Here's the drawing with two shaded views (mm, measured from the low corner). I have some questions. Coordinates: 2 decimals unless noted, no trailing zeros. Write each loop counter-clockwise with the first axis right and the second up, starting at its lowest first coordinate (ties: lowest second). Pieces come first, ordered by that corner, then holes. Notation, with made-up numbers: (58, 63.5) -> (62, 63.5) arc R18 ccw to (62, 92.5) -> close; hole circle Ø7 at (53, -7.75). An arc over 180 degrees is marked (long way). Put each result on its own line as item: value. Start each with the question number.
Item 1: I want a section at A-A, the plane x = 43. List the corners of the cut face in (y, z) for me (1 decimal).
Item 2: If we mould it in two halves opening along X, with no side actions, what happens to the marked faces 1, 2 and 3? For each: released by +X, released by -X, zero draft, split by the parting line, or undercut.
Item 3: I want a section at C-C, the plane z = 16. List the corners of the cut face in (x, y) for me (1 decimal).
Item 4: I need wall thicknesses on line 1 (X direction, y = 2.25, z = 43) (1 decimal); line 2 (Z direction, x = 39.5, y = 0.7) (1 decimal). Which ranges of each line are inside material? Lowest first, please. Write a range as [from, to].
Item 5: I want a section at B-B, the plane z = 43. List the corners of the cut face in (x, y) for me (1 decimal).
Item 6: I want a section at D-D, the plane x = 61. List the corners of the cut face in (y, z) for me (1 decimal), then the cut area to 3 significant figures.
Item 7: For pin 1 (1.6 mm diameter, centred on x = 50, y = 1.5, fed in from -Z); pin 2 (5 mm diameter, centred on x = 73.5, z = 28, fed in from +Y), each with a flat end and sliding along its axis, tell me the tip position at first contact or that it passes through.
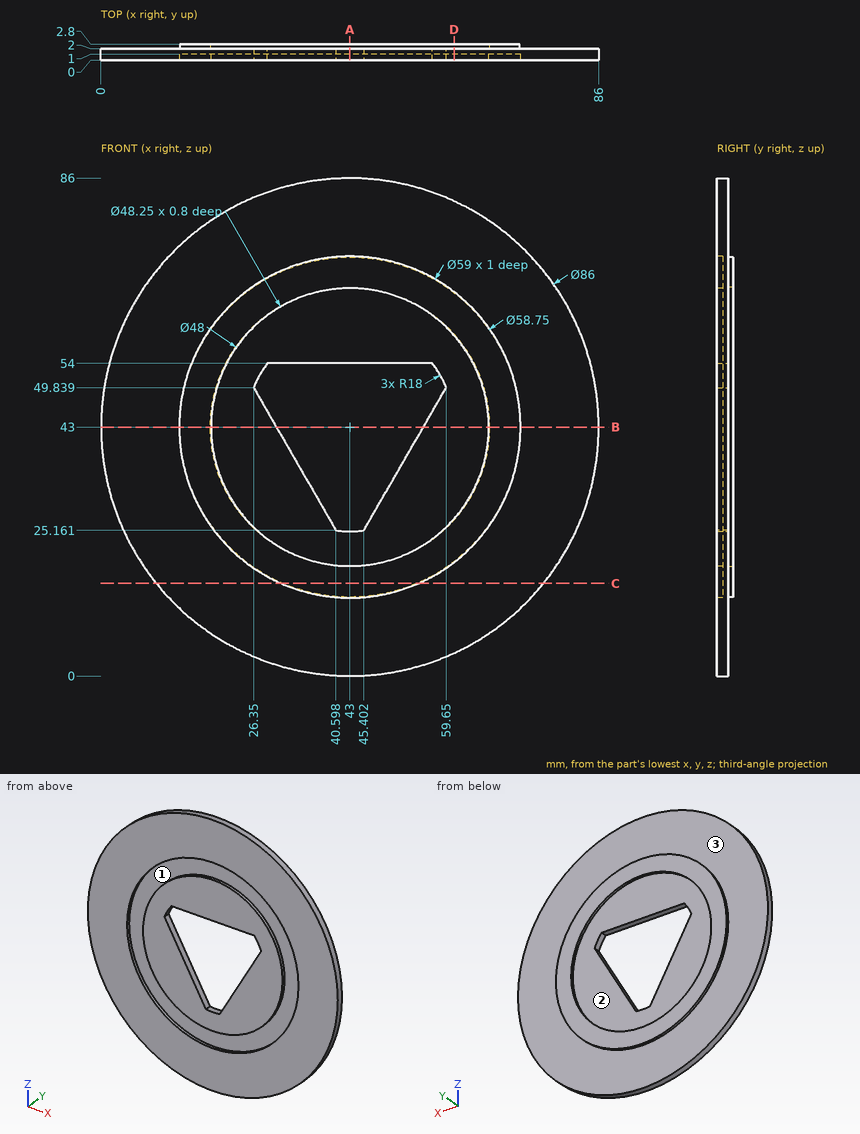
Calculated:
1. outline: (0, 0) -> (2, 0) -> (2, 13.6) -> (2.8, 13.6) -> (2.8, 18.9) -> (2, 18.9) -> (2, 25) -> (0, 25) -> (0, 19) -> (1, 19) -> (1, 13.5) -> (0, 13.5) -> close; (0, 54) -> (2, 54) -> (2, 67.1) -> (2.8, 67.1) -> (2.8, 72.4) -> (2, 72.4) -> (2, 86) -> (0, 86) -> (0, 72.5) -> (1, 72.5) -> (1, 67) -> (0, 67) -> close
2. face 1: undercut
2. face 2: undercut
2. face 3: zero draft
3. outline: (9.5, 0) -> (31.1, 0) -> (31.1, 1) -> (54.9, 1) -> (54.9, 0) -> (76.5, 0) -> (76.5, 2) -> (54.6, 2) -> (54.6, 2.8) -> (31.4, 2.8) -> (31.4, 2) -> (9.5, 2) -> close
4. line 1: x = [13.6, 18.9], [67.1, 72.4]
4. line 2: z = [0.1, 13.7], [19.3, 27.1], [54, 66.7], [72.3, 85.9]
5. outline: (0, 0) -> (13.5, 0) -> (13.5, 1) -> (19, 1) -> (19, 0) -> (30.3, 0) -> (30.3, 2) -> (18.9, 2) -> (18.9, 2.8) -> (13.6, 2.8) -> (13.6, 2) -> (0, 2) -> close; (55.7, 0) -> (67, 0) -> (67, 1) -> (72.5, 1) -> (72.5, 0) -> (86, 0) -> (86, 2) -> (72.4, 2) -> (72.4, 2.8) -> (67.1, 2.8) -> (67.1, 2) -> (55.7, 2) -> close
6. outline: (0, 3.9) -> (2, 3.9) -> (2, 19.8) -> (2.8, 19.8) -> (2.8, 26.9) -> (2, 26.9) -> (2, 59.1) -> (2.8, 59.1) -> (2.8, 66.2) -> (2, 66.2) -> (2, 82.1) -> (0, 82.1) -> (0, 66.4) -> (1, 66.4) -> (1, 58.9) -> (0, 58.9) -> (0, 27.1) -> (1, 27.1) -> (1, 19.6) -> (0, 19.6) -> close
6. area: 153 mm2
7. pin 1: stops at z = 0.45
7. pin 2: stops at y = 2
